The model under review builds one solid part; all positions refer to its coordinate system, in mm. A direction names the side the tool comes from. Give positions to 0.01 mm unless a question says otherwise; leave off trailing zeros. Loops run counter-clockwise (first coordinate to the right, second up) from the corner with the lowest first, then second, coordinate; pieces in that order, holes last. Notation, with made-up numbers: M 34.5,61.25 L 69.5,61.25 A12 cw 69.5,76.25 Z; hole C 80,-2.75 d10. An arc over 180 degrees is marked long. Write item = value, one per line. Start each with the question number.
1. For faces 1 (the face through (14.531, 6.507, -15.846)), 2 (the face through (-10.648, 3.458, -13.887)), 3 (the face through (17.4, 1, 9.5)), list the 3-axis set-ups (+Z, -Z, +X, -X, +Y, -Y) from which the entire face can be reached by the end or side of a thin tool; tool diameter is ignored.
2. Wall thickness on line 1 along X through (y, z) = (6.5, 0); line 2 along Z through (x, y) = (-5, 6.25); line 3 along X through (y, z) = (5, 0): over which ranges is each line inside the solid? List them lowest first. Write a range as from..to.
3. We need section C-C on y = 5. Give the boundary of the cut face in (x, z), then the cut area to 3 significant figures.
4. Draft analysis for pull direction Z (two halves, no side actions). For faces 4 (the face through (-14.531, 0.507, -15.846)), 5 (the face through (15.88, 3.46, -17.32)), 6 (the face through (-17.24, 0, 5.69)), state which applies: pulls with the +Z half, pulls with the -Z half, needs draft (parallel to the pull), parting line crosses it, or undercut.
from build123d import *

# Parameters (mm, degrees)
SKETCH1_R           = 23.5
SKETCH1_R_2         = 17.5
BOSS_EXTRUDE1_DEPTH = 7
SKETCH2_R           = 21.5
SKETCH2_R_2         = 19.5
CUT_EXTRUDE1_DEPTH  = 1
CUT_EXTRUDE2_START  = -1
SKETCH3_R           = 21.5
SKETCH3_R_2         = 19.5
CUT_EXTRUDE2_DEPTH  = 1
CHAMFER1_SIZE       = 0.5


with BuildPart() as part:
    # Sketch1 → Boss-Extrude1 (new body)
    with BuildSketch(Plane(origin=(0, 0, 0), x_dir=(1, 0, 0), z_dir=(0, 1, 0))):
        with Locations(Location((0, 0, 0), (0, 0, 270))):
            Circle(SKETCH1_R)
        with Locations(Location((0, 0, 0), (0, 0, 270))):
            Circle(SKETCH1_R_2, mode=Mode.SUBTRACT)
    extrude(amount=BOSS_EXTRUDE1_DEPTH)

    # Sketch2 → Cut-Extrude1 (cut)
    with BuildSketch(Plane(origin=(0, 7, 0), x_dir=(1, 0, 0), z_dir=(0, 1, 0))):
        with Locations(Location((0, 0, 0), (0, 0, 270))):
            Circle(SKETCH2_R)
        with Locations(Location((0, 0, 0), (0, 0, 270))):
            Circle(SKETCH2_R_2, mode=Mode.SUBTRACT)
    extrude(amount=-CUT_EXTRUDE1_DEPTH, mode=Mode.SUBTRACT)

    # Sketch3 → Cut-Extrude2 (cut)
    with BuildSketch(Plane.XZ.offset(CUT_EXTRUDE2_START)):
        with Locations(Location((0, 0, 0), (0, 0, 90))):
            Circle(SKETCH3_R)
        with Locations(Location((0, 0, 0), (0, 0, 90))):
            Circle(SKETCH3_R_2, mode=Mode.SUBTRACT)
    extrude(amount=CUT_EXTRUDE2_DEPTH, mode=Mode.SUBTRACT)

    # Chamfer1
    chamfer1_edges = [part.edges().sort_by_distance(p)[0] for p in [
        (0, 0, -23.5),
        (0, 7, -23.5),
        (0, 0, -17.5),
        (0, 7, -17.5),
    ]]
    chamfer(chamfer1_edges, length=CHAMFER1_SIZE)


solid = part.part
Final values:
q1.face_1 = +Y
q1.face_2 = +Y, -Y
q1.face_3 = -Y
q2.line_1 = -23.5..-21.5, -19.5..-17.5, 17.5..19.5, 21.5..23.5
q2.line_2 = -22.96..-20.91, -18.85..-16.77, 16.77..18.85, 20.91..22.96
q2.line_3 = -23.5..-17.5, 17.5..23.5
q3.outline = C 0,0 d47; hole C 0,0 d35
q3.area = 773 mm²
q4.face_4 = undercut
q4.face_5 = parting line crosses it
q4.face_6 = needs draft
